```python
from build123d import *

# Parameters (mm, degrees)
BOSS_EXTRUDE1_DEPTH = 10
SKETCH4_W           = 10
SKETCH4_H           = 10
SKETCH4_R           = 3.5
CUT_EXTRUDE8_DEPTH  = 20
SKETCH12_W          = 10
SKETCH12_H          = 10
SKETCH12_R          = 3.5
CUT_EXTRUDE10_DEPTH = 20
SKETCH14_W          = 10
SKETCH14_H          = 10
SKETCH14_R          = 3.5
CUT_EXTRUDE12_DEPTH = 40
BOSS_EXTRUDE2_START = 20
SKETCH15_R          = 3.5
BOSS_EXTRUDE2_DEPTH = 20
SKETCH16_W          = 50
SKETCH16_H          = 20
CUT_EXTRUDE14_DEPTH = 200


with BuildPart() as part:
    # Sketch1 → Boss-Extrude1 (new body)
    with BuildSketch(Plane.XY):
        Polygon((-66, 0), (0, 0), (0, -10), (-43, -10), (-43, -30), (-206, -30), (-206, -10), (-246, -10), (-246, 0), (-196, 0), (-196, -20), (-66, -20), align=None)
    extrude(amount=BOSS_EXTRUDE1_DEPTH)

    # Sketch4 → Cut-Extrude8 (cut, symmetric)
    with BuildSketch(Plane(origin=(0, 0, 0), x_dir=(0, 0, -1), z_dir=(1, 0, 0))):
        with Locations((-5, -5)):
            Rectangle(SKETCH4_W, SKETCH4_H)
        with Locations((-5, -5)):
            Circle(SKETCH4_R, mode=Mode.SUBTRACT)
    extrude(amount=CUT_EXTRUDE8_DEPTH, both=True, mode=Mode.SUBTRACT)

    # Sketch12 → Cut-Extrude10 (cut, symmetric)
    with BuildSketch(Plane(origin=(-131, 0, 0), x_dir=(0, 0, -1), z_dir=(1, 0, 0))):
        with Locations((-5, -25)):
            Rectangle(SKETCH12_W, SKETCH12_H)
        with Locations((-5, -25)):
            Circle(SKETCH12_R, mode=Mode.SUBTRACT)
    extrude(amount=CUT_EXTRUDE10_DEPTH, both=True, mode=Mode.SUBTRACT)

    # Sketch14 → Cut-Extrude12 (cut)
    with BuildSketch(Plane.ZY.offset(246)):
        with Locations((5, -5)):
            Rectangle(SKETCH14_W, SKETCH14_H)
        with Locations(Location((5, -5, 0), (0, 0, 180))):
            Circle(SKETCH14_R, mode=Mode.SUBTRACT)
    extrude(amount=-CUT_EXTRUDE12_DEPTH, mode=Mode.SUBTRACT)

    # Sketch15 → Boss-Extrude2 (add)
    with BuildSketch(Plane.ZY.offset(206).offset(BOSS_EXTRUDE2_START)):
        with Locations(Location((5, -25, 0), (0, 0, 180))):
            Circle(SKETCH15_R)
    extrude(amount=-BOSS_EXTRUDE2_DEPTH)

    # Sketch16 → Cut-Extrude14 (cut)
    with BuildSketch(Plane.XY):
        with Locations((-221, -10)):
            Rectangle(SKETCH16_W, SKETCH16_H)
    extrude(amount=CUT_EXTRUDE14_DEPTH, mode=Mode.SUBTRACT)


solid = part.part
```
Verification items for the finished model (mm, model axes). A direction names the side the tool comes from. Coordinates: 2 decimals unless noted, no trailing zeros. Loops run counter-clockwise (first coordinate to the right, second up) from the corner with the lowest first, then second, coordinate; pieces in that order, holes last. Notation, with made-up numbers: (21, 12.5) - (51, 12.5) arc R34 cw to (51, 43.5) - close; hole circle Ø9 at (8.25, -35). An arc over 180 degrees is marked (long way). Return JSON: item names as keys, results as strings.
1. Section check A-A, the plane z = 5. Record the boundary of the cut face in (x, y).
Established:
{"outline": "(-226, -28.5) - (-206, -28.5) - (-206, -30) - (-151, -30) - (-151, -28.5) - (-111, -28.5) - (-111, -30) - (-43, -30) - (-43, -10) - (-20, -10) - (-20, -8.5) - (0, -8.5) - (0, -1.5) - (-20, -1.5) - (-20, 0) - (-66, 0) - (-66, -20) - (-111, -20) - (-111, -21.5) - (-151, -21.5) - (-151, -20) - (-206, -20) - (-206, -21.5) - (-226, -21.5) - close"}
2. Tool access check on faces 5 (the flat face through (-178, -25, 0)), 6 (the flat face through (-31, -10, 5)), 7 (the cylindrical face through (-10.14, -6.341, 1.767)), 8 (the flat face through (-151, -22.7, 8.4)), 9 (the flat face through (-179, -20, 5)). Record the directions out of +Z, -Z, +X, -X, +Y, -Y that give a thin tool (end or side, any length) a straight path to the whole face; none if there is none.
Established:
{"face 5": "-Z, +X, -X, +Y, -Y", "face 6": "+Z, -Z, +X, -Y", "face 7": "+X", "face 8": "none", "face 9": "+Z, -Z, -X, +Y"}
3. Section check B-B, the plane y = -5. Record the boundary of the cut face in (x, z), then the cut area to 3 significant figures.
Established:
{"outline": "(-66, 0) - (-20, 0) - (-20, 1.5) - (0, 1.5) - (0, 8.5) - (-20, 8.5) - (-20, 10) - (-66, 10) - close", "area": "600 mm2"}
4. Mould release check, pull along X, two halves, no side actions. Record for faces 1 (the cylindrical face through (-131.28, -21.53, 5.46)), 2 (the flat face through (-206, -22.7, 1.6)), 3 (the flat face through (-111, -22.7, 8.4)), 4 (the flat face through (-65, -15, 10)): +X half, -X half, draft (parallel to the pull), parting line (faces both ways), or undercut.
Established:
{"face 1": "undercut", "face 2": "-X half", "face 3": "undercut", "face 4": "draft"}
5. Go/stop test with flat-tipped pins: pin 1 (3 mm diameter, centred on x = -33.5, z = 5.5, fed in from -Y); pin 2 (4 mm diameter, centred on y = -11.5, z = 7, fed in from -X); pin 3 (5 mm diameter, centred on x = -88.5, z = 6, fed in from +Y). Record where each tip stops, or that it passes through.
Established:
{"pin 1": "stops at y = -10", "pin 2": "stops at x = -66", "pin 3": "stops at y = -20"}
6. Section check C-C, the plane x = -116.5. Record the boundary of the cut face in (y, z).
Established:
{"outline": "circle Ø7 at (-25, 5)"}
7. Thickness scan on L1, parallel to X at y = -24.5, z = 8.75; L2, parallel to Y at x = -113.5, z = 5.5; L3, parallel to X at y = -5, z = 3.5. Record the ranges inside material, lowest first.
Established:
{"L1": "x = -206 to -151, -111 to -43", "L2": "y = -28.46 to -21.54", "L3": "x = -66 to 0"}
8. Section check D-D, the plane y = -25. Record the boundary of the cut face in (x, z), then the cut area to 3 significant figures.
Established:
{"outline": "(-226, 1.5) - (-206, 1.5) - (-206, 0) - (-151, 0) - (-151, 1.5) - (-111, 1.5) - (-111, 0) - (-43, 0) - (-43, 10) - (-111, 10) - (-111, 8.5) - (-151, 8.5) - (-151, 10) - (-206, 10) - (-206, 8.5) - (-226, 8.5) - close", "area": "1,650 mm2"}
